Geometry: final body of the model. Coordinates: model frame, mm. Face numbers are marked on the shaded views. A direction names the side the tool comes from. Give positions to 0.01 mm unless a question says otherwise; leave off trailing zeros. Write each loop counter-clockwise with the first axis right and the second up, starting at its lowest first coordinate (ties: lowest second). Pieces come first, ordered by that corner, then holes.
Q1. Section C-C (y = -7). Return the cut outline in (x, z).
Q2. Line query: line 1 (Y direction, x = 8.5, z = -8.5); line 2 (Y direction, x = -3.5, z = 3); line 3 (X direction, y = -11.25, z = 1.5). Output: solid intervals per line, ascending.
Q3. Section D-D (z = 10.75). Return the cut outline in (x, y).
Q4. Pin query (flat end, axial travel): pin 1 Ø2 at (x, y) = (-4.5, -14) entering from +Z; pin 2 Ø4 at (x, y) = (7.5, -11) entering from -Z; pin 3 Ø1 at (y, z) = (-16, 0.5) entering from +X; pin 4 Ø3 at (x, y) = (3.5, -16) entering from +Z. Return the tip coordinate at first contact, or that it passes through.
Q5. Section B-B (x = 0). Return the cut outline in (y, z).
Q6. Section A-A (z = 0). Return the cut outline in (x, y).
Q7. Reachability of the marked faces 1 and 2 from +Z, -Z, +X, -X, +Y, -Y: full face, straight path, thin tool, end or side. Return the list, or none.
from build123d import *

# Parameters (mm, degrees)
SKETCH1_R           = 12.7
BOSS_EXTRUDE1_DEPTH = 2.54
SKETCH3_R           = 5.08
BOSS_EXTRUDE2_DEPTH = 15.24


with BuildPart() as part:
    # Sketch1 → Boss-Extrude1 (new body)
    with BuildSketch(Plane(origin=(0, 0, 0), x_dir=(1, 0, 0), z_dir=(0, 1, 0))):
        with Locations(Location((0, 0, 0), (0, 0, 270))):
            Circle(SKETCH1_R)
    extrude(amount=BOSS_EXTRUDE1_DEPTH)

    # Sketch3 → Boss-Extrude2 (add)
    with BuildSketch(Plane.XZ):
        with Locations(Location((0, 0, 0), (0, 0, 90))):
            Circle(SKETCH3_R)
    extrude(amount=BOSS_EXTRUDE2_DEPTH)

    # Sketch5 → Revolve2 (revolve)
    with BuildSketch(Plane(origin=(0, 0, 0), x_dir=(0, 0, -1), z_dir=(1, 0, 0))):
        with BuildLine():
            Line((0, -15.24), (0, -20.32))
            ThreePointArc((0, -20.32), (-3.592102448, -18.832102448), (-5.08, -15.24))
            Line((-5.08, -15.24), (0, -15.24))
        make_face()
    revolve(axis=Axis((0, -15.24, 0), (0, -1, 0)))


solid = part.part
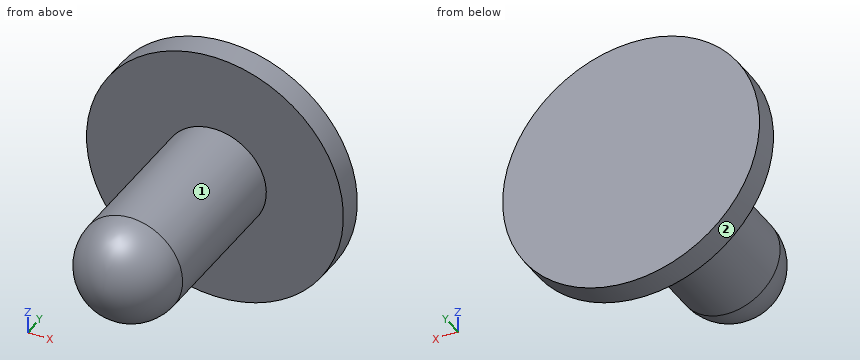
Computed:
1. outline: circle Ø10.16 at (0, 0)
2. line 1: y = 0 to 2.54
2. line 2: y = -17.37 to 2.54
2. line 3: x = -4.85 to 4.85
3. outline: (-6.76, 0) - (6.76, 0) - (6.76, 2.54) - (-6.76, 2.54) - close
4. pin 1: stops at z = 3.68
4. pin 2: passes through
4. pin 3: stops at x = 5.06
4. pin 4: stops at z = 4.63
5. outline: (-15.24, -5.08) - (0, -5.08) - (0, -12.7) - (2.54, -12.7) - (2.54, 12.7) - (0, 12.7) - (0, 5.08) - (-15.24, 5.08) arc R5.08 ccw to start
6. outline: (-12.7, 0) - (-5.08, 0) - (-5.08, -15.24) arc R5.08 ccw to (5.08, -15.24) - (5.08, 0) - (12.7, 0) - (12.7, 2.54) - (-12.7, 2.54) - close
7. face 1: -Y
7. face 2: +Y, -Y
